```python
from build123d import *

# Parameters (mm, degrees)
F0_R      = 25
F1_DEPTH  = 50
F2_R      = 5
F3_W      = 100
F3_H      = 10
F4_DEPTH  = 10
F5_R      = 4.99999
F6_R      = 4
F7_DEPTH  = 10
F8_DEPTH  = 10
F10_DEPTH = 40
F11_R     = 5


# Not quite as in the source:
# - a fillet or chamfer is up to 0.001 mm smaller than in the source, because OpenCascade refuses the exact size


with BuildPart() as f1:
    # F0 (on Top) → F1 (new body)
    with BuildSketch(Plane.XY):
        Circle(F0_R)
    extrude(amount=F1_DEPTH)

    # F2
    f2_edges = [f1.edges().sort_by_distance(p)[0] for p in [
        (-25, 0, 50),
    ]]
    fillet(f2_edges, radius=F2_R)

    # F3 (on face) → F4 (join)
    with BuildSketch(Plane(origin=(0, 0, 0), x_dir=(1, 0, 0), z_dir=(0, 0, -1))):
        Rectangle(F3_W, F3_H)
    extrude(amount=F4_DEPTH)

    # F5 (radius 5 in the source; OpenCascade refuses exactly that, so slightly less here)
    f5_edges = [f1.edges().sort_by_distance(p)[0] for p in [
        (-50, 5, -5),
        (-50, -5, -5),
        (50, -5, -5),
        (50, 5, -5),
    ]]
    fillet(f5_edges, radius=F5_R)

    # F6 (on face) → F7 (join)
    with BuildSketch(Plane.XY):
        with Locations((-45, 0)):
            Circle(F6_R)
        with Locations((45, 0)):
            Circle(F6_R)
    extrude(amount=F7_DEPTH)

    # F8 (add): faces of the model
    f8_faces = [f1.faces().sort_by_distance(p)[0] for p in [
        (0, -13.3591920493, 0),
        (0, 13.3591920493, 0),
    ]]
    extrude(f8_faces, amount=F8_DEPTH)

    # F9 (on face) → F10 (cut)
    with BuildSketch(Plane(origin=(0, 0, -10), x_dir=(1, 0, 0), z_dir=(0, 0, -1))):
        Polygon((1.575, 2.7279800219), (-1.575, 2.7279800219), (-3.15, 0), (-1.575, -2.7279800219), (1.575, -2.7279800219), (3.15, 0), align=None)
    extrude(amount=-F10_DEPTH, mode=Mode.SUBTRACT)

    # F11
    f11_edges = [f1.edges().sort_by_distance(p)[0] for p in [
        (23.535534, 0, 48.535534),
        (-25, 0, 45),
        (-20, 0, 50),
        (24.494897, 5, -5),
        (24.494897, -5, -5),
        (-24.494897, -5, -5),
        (-24.494897, 5, -5),
    ]]
    fillet(f11_edges, radius=F11_R)


solid = f1.part
```
Model file for the job. Use its own axes, mm. A direction names the side the tool comes from. Coordinates: 2 decimals unless noted, no trailing zeros. Order: outer loops, then holes, each group sorted by start corner. A loop starts at its lowest first (then second) coordinate and runs counter-clockwise, first axis right, second up. Notation, with made-up numbers: (-36, -7.75) -> (-9, -7.75) arc R35 cw to (-9, 25.25) -> close; hole circle Ø7 at (-18.75, 4). An arc over 180 degrees is marked (long way). Return JSON: item names as keys, results as strings.
Item 1: Pin check, flat tips, straight feed: P1, Ø2.5, axis at x = 43.5, y = -1.5, coming from the +Z side; P2, Ø1.6, axis at x = 0.5, z = 9.5, coming from the -Y side; P3, Ø11, axis at x = -35, z = -7, coming from the +Y side. Stop position of each tip, or through.
Model answer:
{"P1": "stops at z = 10", "P2": "stops at y = -25", "P3": "stops at y = 5"}
Item 2: 3-axis set-ups, long thin cutter, end or side, ignore diameter. For faces 4 (the face through (11.5, -22.2, 17.9)), 5 (the face through (2.351, 1.383, 9.72)), 6 (the face through (-37, 5, -5)), 7 (the face through (37, 5, -5)): which of +Z, -Z, +X, -X, +Y, -Y reach the whole face in a straight line?
Model answer:
{"face 4": "+Z", "face 5": "-Z", "face 6": "+Z, -Z, -X, +Y", "face 7": "+Z, -Z, +X, +Y"}
Item 3: Mould opens along X. For faces 1 (the face through (0, 0, 50)), 2 (the face through (41.8, -2.4, 4.9)), 3 (the face through (-25.362, -5.943, -5.07)) say: pulls with the +X half, pulls with the -X half, needs draft (parallel to the pull), parting line crosses it, or undercut.
Model answer:
{"face 1": "needs draft", "face 2": "undercut", "face 3": "pulls with the -X half"}
Item 4: Wall check: line 1 along Y through (x, z) = (-15, 16); line 2 along Y through (x, z) = (-17.5, -3); line 3 along Z through (x, y) = (-41.5, -4). Give the ranges that are in metal, low to high. Write a range as from..to.
Model answer:
{"line 1": "y = -20..20", "line 2": "y = -17.85..17.85", "line 3": "z = -10..0"}
Item 5: Slice it at B-B (z = 18.5). Write the cut outline in (x, y) (3 decimals).
Model answer:
{"outline": "circle Ø50 at (0, 0); hole (-3.15, 0) -> (-1.575, -2.728) -> (1.575, -2.728) -> (3.15, 0) -> (1.575, 2.728) -> (-1.575, 2.728) -> close"}
Item 6: Slice it at A-A (x = 0). Write the cut outline in (y, z).
Model answer:
{"outline": "(-25, -10) -> (-2.73, -10) -> (-2.73, 30) -> (2.73, 30) -> (2.73, -10) -> (25, -10) -> (25, 45) arc R5 ccw to (20, 50) -> (-20, 50) arc R5 ccw to (-25, 45) -> close"}
Item 7: Slice it at C-C (z = 34.5). Write the cut outline in (x, y).
Model answer:
{"outline": "circle Ø50 at (0, 0)"}
